The model under review builds one solid part; all positions refer to its coordinate system, in mm. A direction names the side the tool comes from. Round coordinates to 2 decimals unless told otherwise and drop trailing zeros. Write each loop counter-clockwise with the first axis right and the second up, starting at its lowest first coordinate (ties: lowest second). Pieces come first, ordered by that corner, then holes. Notation, with made-up numbers: (84.5, 59) -> (89.5, 59) arc R24 ccw to (89.5, 70) -> close; hole circle Ø3 at (47, 71). An arc over 180 degrees is marked (long way). Return JSON: item names as keys, results as strings. Group by question number.
1. Tool access review of faces 1 (the flat face through (0, -5, 32)), 2 (the cylindrical face through (30, -2, 0)): name each direction out of +Z, -Z, +X, -X, +Y, -Y from which nothing blocks a thin tool from reaching the whole face with its end or side.
2. Take a section at D-D, the plane z = 32.5. Write out the cut boundary in (x, y).
3. Take a section at C-C, the plane x = -5. Write out the cut boundary in (y, z).
4. Clearance check with flat-ended pins moving along their axes: P1, Ø1.5, axis at y = -2.5, z = -3.5, coming from the -X side; P2, Ø1, axis at x = -10.5, y = 0.5, coming from the +Z side; P3, Ø10, axis at x = 31.5, z = -15, coming from the -Y side; P4, Ø2, axis at x = 29.5, y = 0, coming from the -Z side. State where each tip first meets the part, or that it passes through.
5. Mouldability with a two-part tool opening along X and no side actions: class faces 3 (the cylindrical face through (-26.547, 1.014, -26.486)), 4 (the cylindrical face through (0, -2, -35)), 5 (the flat face through (32, -5, 0)) as pulls with the +X half, pulls with the -X half, needs draft (parallel to the pull), parting line crosses it, or undercut.
6. For line 1 along X through (y, z) = (0.9, 0); line 2 along X through (y, z) = (-1.75, -1); line 3 along Z through (x, y) = (-9.5, 0.75), list the stretches that pass through material, from the lowest coordinate up. Write a range as from..to.
7. Take a section at B-B, the plane y = -3.75. Write out the cut boundary in (x, z), then the cut area to 3 significant figures.
8. Take a section at A-A, the plane z = 24. Write out the cut boundary in (x, y), then the cut area to 3 significant figures.
from build123d import *

# Parameters (mm, degrees)
SKETCH2_R           = 40
SKETCH2_R_2         = 25
BOSS_EXTRUDE2_DEPTH = 2
SKETCH4_R           = 2.5
BOSS_EXTRUDE3_DEPTH = 5
SKETCH5_R           = 2.5
CUT_EXTRUDE1_DEPTH  = 10
FILLET1_R           = 1
FILLET2_R           = 1


with BuildPart() as part:
    # Sketch2 → Boss-Extrude2 (new body)
    with BuildSketch(Plane(origin=(0, 0, 0), x_dir=(1, 0, 0), z_dir=(0, 1, 0))):
        with Locations(Location((0, 0, 0), (0, 0, 270))):
            Circle(SKETCH2_R)
        with Locations(Location((0, 0, 0), (0, 0, 270))):
            Circle(SKETCH2_R_2, mode=Mode.SUBTRACT)
    extrude(amount=BOSS_EXTRUDE2_DEPTH)

    # Sketch4 → Boss-Extrude3 (add)
    with BuildSketch(Plane.XZ):
        with Locations(Location((0, -32.5, 0), (0, 0, 90))):
            Circle(SKETCH4_R)
        with Locations(Location((32.5, 0, 0), (0, 0, 90))):
            Circle(SKETCH4_R)
        with Locations(Location((0, 32.5, 0), (0, 0, 90))):
            Circle(SKETCH4_R)
        with Locations(Location((-32.5, 0, 0), (0, 0, 90))):
            Circle(SKETCH4_R)
    extrude(amount=BOSS_EXTRUDE3_DEPTH)

    # Sketch5 → Cut-Extrude1 (cut)
    with BuildSketch(Plane(origin=(0, 2, 0), x_dir=(1, 0, 0), z_dir=(0, 1, 0))):
        with Locations((-28.284271247, 28.284271247)):
            Circle(SKETCH5_R)
    extrude(amount=-CUT_EXTRUDE1_DEPTH, mode=Mode.SUBTRACT)

    # Fillet1
    fillet1_edges = [part.edges().sort_by_distance(p)[0] for p in [
        (-26.462124956, 1, -29.995932105),
    ]]
    fillet(fillet1_edges, radius=FILLET1_R)

    # Fillet2
    fillet2_edges = [part.edges().sort_by_distance(p)[0] for p in [
        (-29.995932105, 1, -26.462124956),
    ]]
    fillet(fillet2_edges, radius=FILLET2_R)


solid = part.part
Output:
{
 "1": {"face 1": "+Z, -Z, +X, -X, -Y", "face 2": "-Y"},
 "2": {"outline": "(-23.32, 0) -> (-2.5, 0) -> (-2.5, -5) -> (2.5, -5) -> (2.5, 0) -> (23.32, 0) -> (23.32, 2) -> (-23.32, 2) -> close"},
 "3": {"outline": "(0, -39.69) -> (2, -39.69) -> (2, -24.49) -> (0, -24.49) -> close; (0, 24.49) -> (2, 24.49) -> (2, 39.69) -> (0, 39.69) -> close"},
 "4": {"P1": "passes through", "P2": "stops at z = 38.73", "P3": "stops at y = 0", "P4": "stops at z = -28.07"},
 "5": {"face 3": "undercut", "face 4": "parting line crosses it", "face 5": "needs draft"},
 "6": {"line 1": "x = -40..-25, 25..40", "line 2": "x = -34.79..-30.21, 30.21..34.79", "line 3": "z = -38.86..-23.12, 23.12..38.86"},
 "7": {"outline": "circle Ø5 at (-32.5, 0); circle Ø5 at (0, -32.5); circle Ø5 at (0, 32.5); circle Ø5 at (32.5, 0)", "area": "78.5 mm^2"},
 "8": {"outline": "(-32, 0) -> (-7, 0) -> (-7, 2) -> (-32, 2) -> close; (7, 0) -> (32, 0) -> (32, 2) -> (7, 2) -> close", "area": "100 mm^2"}
}
